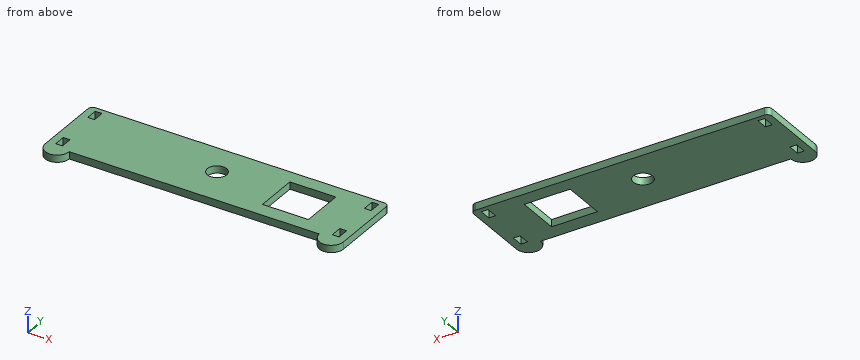
Autodesk Inventor part; units mm, degrees
ref_plane "YZ Plane" through (0, 0, 0) normal (1, 0, 0) x (0, 1, 0)
ref_plane "XZ Plane" through (0, 0, 0) normal (0, 1, 0) x (-1, 0, 0)
ref_plane "XY Plane" through (0, 0, 0) normal (0, 0, 1) x (1, 0, 0)
sketch "Sketch1" plane through (0, 0, 0) normal (0, 0, 1) x (1, 0, 0)
  line L0 (-62, 15) -> (62, 15)
  line L1 (62, 15) -> (62, -15)
  line L2 (62, -15) -> (-62, -15)
  line L3 (-62, -15) -> (-62, 15)
  line L4 (-62, 15) -> (62, -15) construction
  line L5 (62, 15) -> (-62, -15) construction
  point P0 (0, 0)
  dimension "d0" = 124
  dimension "d1" = 30
extrude "Extrusion1" add sketch "Sketch1" along normal blind 3
sketch "Sketch3" plane through (0, 0, 3) normal (0, 0, 1) x (1, 0, 0)
  line L0 (62, 15) -> (-62, 15)
  line L1 (-62, -15) -> (62, -15)
  arc A0 (-62, -15) -> (-52, -15) centre (-57, -15) ccw
  line L2 (-62, -15) -> (-52, -15)
  point P0 (0, 0)
extrude "Extrusion3" add sketch "Sketch3" against normal blind 3
mirror "Mirror2" about plane through (0, 0, 0) normal (1, 0, 0) of "Extrusion3"
fillet "Fillet1" radius 2 1 edges at (-62, 15, 1.5)
fillet "Fillet2" radius 2 1 edges at (62, 15, 1.5)
sketch "Sketch5" plane through (0, 0, 3) normal (0, 0, 1) x (1, 0, 0)
  line L0 (-58.91, 12.96) -> (-56.09, 12.96)
  line L1 (-56.09, 12.96) -> (-56.09, 8.04)
  line L2 (-56.09, 8.04) -> (-58.91, 8.04)
  line L3 (-58.91, 8.04) -> (-58.91, 12.96)
  line L4 (-58.91, 12.96) -> (-56.09, 8.04) construction
  line L5 (-56.09, 12.96) -> (-58.91, 8.04) construction
  line L6 (60, 15) -> (-60, 15)
  line L7 (-58.91, -8.04) -> (-56.09, -8.04)
  line L8 (-56.09, -8.04) -> (-56.09, -12.96)
  line L9 (-56.09, -12.96) -> (-58.91, -12.96)
  line L10 (-58.91, -12.96) -> (-58.91, -8.04)
  line L11 (-58.91, -8.04) -> (-56.09, -12.96) construction
  line L12 (-56.09, -8.04) -> (-58.91, -12.96) construction
  line L13 (-52, -15) -> (52, -15)
  point P0 (0, 0)
  point P1 (-57.5, 10.5)
  point P2 (-57.5, -10.5)
  point P3 (-57.5, -10.5)
  point P4 (-57.5, 10.5)
  dimension "d31" = 2.82
  dimension "d32" = 4.92
  dimension "d33" = 57.5
  dimension "d34" = 4.5
  dimension "d35" = 4.5
extrude "Extrusion5" cut sketch "Sketch5" against normal through all
mirror "Mirror3" about plane through (0, 0, 0) normal (1, 0, 0) of "Extrusion5"
sketch "Sketch4" plane through (0, 0, 3) normal (0, 0, 1) x (1, 0, 0)
  line L0 (24.4, 9.2) -> (43.5, 9.2)
  line L1 (43.5, 9.2) -> (43.5, -8.8)
  line L2 (43.5, -8.8) -> (24.4, -8.8)
  line L3 (24.4, -8.8) -> (24.4, 9.2)
  circle A0 centre (-0.9, 1.3) radius 4
  line L4 (62, -15) -> (62, 13)
  line L5 (-52, -15) -> (52, -15)
  line L6 (48.8866, -5.2) -> (-45.0961, -5.2) construction
  line L7 (-51.0965, -10) -> (52, -10) construction
  line L8 (58.91, -12.96) -> (56.09, -12.96)
  line L9 (56.09, -12.96) -> (56.09, -8.04)
  line L10 (56.09, -8.04) -> (58.91, -8.04)
  line L11 (58.91, -8.04) -> (58.91, -12.96)
  line L12 (56.09, -8.04) -> (58.91, -12.96) construction
  line L13 (56.09, -12.96) -> (58.91, -8.04) construction
  line L14 (60, 15) -> (-60, 15)
  point P0 (0, 0)
  point P1 (57.5, -10.5)
  dimension "d19" = 18
  dimension "d20" = 19.1
  dimension "d24" = 8
  dimension "d28" = 3.6
  dimension "d29" = 5
  dimension "d30" = 4.8
  dimension "d39" = 58.4
  dimension "d41" = 13.7
  dimension "d42" = 18.5
extrude "Extrusion4" cut sketch "Sketch4" against normal through all contours L0 L1 L2 L3 | A0
equation "\"kerf\" = 0.13"
properties part number "FrontPanel" material "Acrylic, Clear"
Input: part model. Units: mm. Frame: model coordinates. Give positions to 0.01 mm unless a question says otherwise; leave off trailing zeros. Order: outer loops, then holes, each group sorted by start corner. A loop starts at its lowest first (then second) coordinate and runs counter-clockwise, first axis right, second up. Notation, with made-up numbers: (20.5, 53) - (29.5, 53) arc R21 ccw to (29.5, 80) - close; hole circle Ø6 at (35.25, 87.5). An arc over 180 degrees is marked (long way). Put each result on its own line as item: value.
Item 1: Section query A-A, the plane y = -5.5. Return loops of the section in (x, z).
Found:
outline: (-62, 0) - (24.4, 0) - (24.4, 3) - (-62, 3) - close; (43.5, 0) - (62, 0) - (62, 3) - (43.5, 3) - close
Item 2: Section query B-B, the plane x = 35.5. Return loops of the section in (y, z).
Found:
outline: (-15, 0) - (-8.8, 0) - (-8.8, 3) - (-15, 3) - close; (9.2, 0) - (15, 0) - (15, 3) - (9.2, 3) - close
Item 3: Contact query for a flat-ended pin moving along its axis: pin 1 (1.5 mm diameter, centred on x = -24, z = 1, fed in from -Y). Output: stop coordinate, or through.
Found:
pin 1: stops at y = -15
Item 4: Section query D-D, the plane y = 11. Return loops of the section in (x, z).
Found:
outline: (-62, 0) - (-58.91, 0) - (-58.91, 3) - (-62, 3) - close; (-56.09, 0) - (56.09, 0) - (56.09, 3) - (-56.09, 3) - close; (58.91, 0) - (62, 0) - (62, 3) - (58.91, 3) - close
Item 5: Section query C-C, the plane z = 1.4. Count the separate pieces of the cut face and the enclosed holes in it, then the cut area to 3 significant figures.
Found:
separate pieces: 1
enclosed holes: 6
area: 3,350 mm^2
Item 6: Ray query, L1, parallel to X at y = 10.5, z = 1.3; L2, parallel to X at y = 8.5, z = 2.8; L3, parallel to Y at x = -57, z = 0.75. Return the intervals inside material, ascending. Write a range as from..to.
Found:
L1: x = -62..-58.91, -56.09..56.09, 58.91..62
L2: x = -62..-58.91, -56.09..24.4, 43.5..56.09, 58.91..62
L3: y = -20..-12.96, -8.04..8.04, 12.96..15
